Geometry check sheet. Reference: the model listing, model coordinates, mm. A direction names the side the tool comes from. Round coordinates to 2 decimals unless told otherwise and drop trailing zeros. Loops run counter-clockwise (first coordinate to the right, second up) from the corner with the lowest first, then second, coordinate; pieces in that order, holes last. Notation, with made-up numbers: (9.25, 60.25) - (32.25, 60.25) arc R14 cw to (32.25, 81.25) - close; hole circle Ø8 at (72, 63). An arc over 180 degrees is marked (long way). Answer as CSV lines item,"result". Start each with the question number.
1) Cross-section at B-B on x = -28. Record the boundary of the cut face in (y, z).
2) Cross-section at C-C on y = 0. Record the boundary of the cut face in (x, z) (3 decimals).
3) Cross-section at D-D on x = -37. Record the boundary of the cut face in (y, z) (3 decimals).
4) Depth check by flat-ended pin: P1, Ø5, axis at x = -8.3, y = -10, coming from the -Z side. Enter the tip coordinate at first touch or a pass-through.
5) Draft check along Y on faces 3 (the flat face through (31, -6, 1)), 4 (the flat face through (37.1, 9.59, 1.01)), 5 (the flat face through (40, 0, 1)), 6 (the cylindrical face through (30.43, -2.6, 0.99)). Enter one of: released by +Y, released by -Y, zero draft, split by the parting line, or undercut.
6) Access from +Z, -Z, +X, -X, +Y, -Y to the whole of each face (thin tool, end or side, straight path). Record for faces 1 (the cylindrical face through (-39.43, 13.9, 1.01)), 2 (the flat face through (13, 2, 1)).
7) Cross-section at A-A on x = 18.5. Record the boundary of the cut face in (y, z), and give its area (3 significant figures).
8) Thickness scan on line 1 along Y through (x, z) = (-8.3, 0.8) (3 decimals); line 2 along X through (y, z) = (3.75, 1.5); line 3 along Y through (x, z) = (6.5, 0.85). Record the ranges inside material, lowest first.
from build123d import *

# Parameters (mm, degrees)
SKETCH_1_W          = 80
SKETCH_1_H          = 29
EXTRUDE_1_DEPTH     = 2
CUT_EXTRUDE_1_DEPTH = 2
SKETCH_3_R          = 1.525
CUT_EXTRUDE_2_DEPTH = 10
SKETCH_4_R          = 1.525
CUT_EXTRUDE_3_DEPTH = 10
FILLET_1_R          = 2
SKETCH_5_W          = 20.7
SKETCH_5_H          = 19
CUT_EXTRUDE_4_DEPTH = 10
SKETCH_6_W          = 35.3
SKETCH_6_H          = 7.5
CUT_EXTRUDE_5_DEPTH = 10
FILLET_2_R          = 2


with BuildPart() as part:
    # 草图1 → 凸台-拉伸1 (new body)
    with BuildSketch(Plane.XY):
        Rectangle(SKETCH_1_W, SKETCH_1_H)
    extrude(amount=EXTRUDE_1_DEPTH)

    # 草图2 → 切除-拉伸1 (cut)
    with BuildSketch(Plane.XY.offset(2)):
        Polygon((34, 14.5), (40, 5), (40, 14.5), align=None)
        Polygon((40, -14.5), (34, -14.5), (40, -5), align=None)
    extrude(amount=-CUT_EXTRUDE_1_DEPTH, mode=Mode.SUBTRACT)

    # 草图3 → 切除-拉伸2 (cut)
    with BuildSketch(Plane.XY.offset(2)):
        with Locations((-8.3, 10)):
            Circle(SKETCH_3_R)
        with Locations((-37, 0)):
            Circle(SKETCH_3_R)
        with Locations((-8.3, -10)):
            Circle(SKETCH_3_R)
    extrude(amount=-CUT_EXTRUDE_2_DEPTH, mode=Mode.SUBTRACT)

    # 草图4 → 切除-拉伸3 (cut)
    with BuildSketch(Plane.XY.offset(2)):
        with Locations((35, 0)):
            Circle(SKETCH_4_R)
    extrude(amount=-CUT_EXTRUDE_3_DEPTH, mode=Mode.SUBTRACT)

    # 圆角1
    fillet_1_edges = [part.edges().sort_by_distance(p)[0] for p in [
        (34, 14.5, 1),
        (40, 5, 1),
        (40, -5, 1),
        (34, -14.5, 1),
        (-40, -14.5, 1),
        (-40, 14.5, 1),
    ]]
    fillet(fillet_1_edges, radius=FILLET_1_R)

    # 草图5 → 切除-拉伸4 (cut)
    with BuildSketch(Plane.XY.offset(2)):
        with Locations((-22.65, 0)):
            Rectangle(SKETCH_5_W, SKETCH_5_H)
    extrude(amount=-CUT_EXTRUDE_4_DEPTH, mode=Mode.SUBTRACT)

    # 草图6 → 切除-拉伸5 (cut)
    with BuildSketch(Plane.XY.offset(2)):
        with Locations((13.35, 5.75)):
            Rectangle(SKETCH_6_W, SKETCH_6_H)
        with Locations((13.35, -5.75)):
            Rectangle(SKETCH_6_W, SKETCH_6_H)
    extrude(amount=-CUT_EXTRUDE_5_DEPTH, mode=Mode.SUBTRACT)

    # 圆角2
    fillet_2_edges = [part.edges().sort_by_distance(p)[0] for p in [
        (-33, 9.5, 1),
        (-12.3, 9.5, 1),
        (-12.3, -9.5, 1),
        (-33, -9.5, 1),
        (-4.3, 2, 1),
        (-4.3, 9.5, 1),
        (31, 9.5, 1),
        (31, 2, 1),
        (-4.3, -2, 1),
        (31, -2, 1),
        (31, -9.5, 1),
        (-4.3, -9.5, 1),
    ]]
    fillet(fillet_2_edges, radius=FILLET_2_R)


solid = part.part
Answer block:
1,outline,"(-14.5, 0) - (-9.5, 0) - (-9.5, 2) - (-14.5, 2) - close; (9.5, 0) - (14.5, 0) - (14.5, 2) - (9.5, 2) - close"
2,outline,"(-40, 0) - (-38.525, 0) - (-38.525, 2) - (-40, 2) - close; (-35.475, 0) - (-33, 0) - (-33, 2) - (-35.475, 2) - close; (-12.3, 0) - (33.475, 0) - (33.475, 2) - (-12.3, 2) - close; (36.525, 0) - (40, 0) - (40, 2) - (36.525, 2) - close"
3,outline,"(-14.5, 0) - (-1.525, 0) - (-1.525, 2) - (-14.5, 2) - close; (1.525, 0) - (14.5, 0) - (14.5, 2) - (1.525, 2) - close"
4,P1,"stops at z = 0"
5,face 3,"undercut"
5,face 4,"released by +Y"
5,face 5,"zero draft"
5,face 6,"undercut"
6,face 1,"+Z, -Z, -X, +Y"
6,face 2,"+Z, -Z"
7,outline,"(-14.5, 0) - (-9.5, 0) - (-9.5, 2) - (-14.5, 2) - close; (-2, 0) - (2, 0) - (2, 2) - (-2, 2) - close; (9.5, 0) - (14.5, 0) - (14.5, 2) - (9.5, 2) - close"
7,area,"28.0 mm^2"
8,line 1,"y = -14.5 to -11.525, -8.475 to 8.475, 11.525 to 14.5"
8,line 2,"x = -40 to -33, -12.3 to -4.28, 30.98 to 40"
8,line 3,"y = -14.5 to -9.5, -2 to 2, 9.5 to 14.5"
